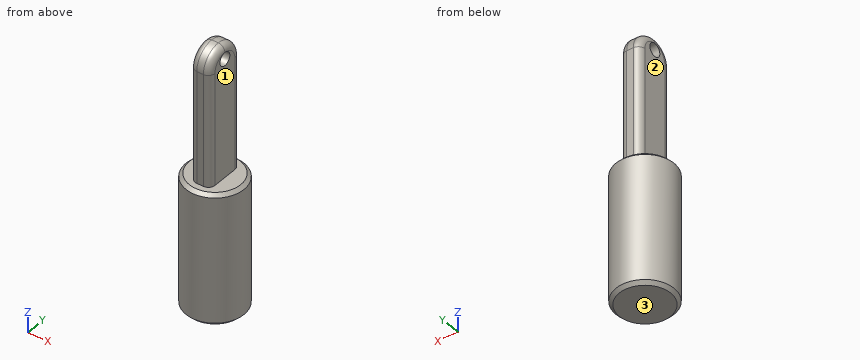
from build123d import *

# Parameters (mm, degrees)
SKETCH2_R           = 22
BOSS_EXTRUDE1_DEPTH = 100
SKETCH4_W           = 100
SKETCH4_H           = 30
BOSS_EXTRUDE2_DEPTH = 7.5
FILLET1_R           = 15
SKETCH5_R           = 5
CUT_EXTRUDE1_DEPTH  = 107.556323135
FILLET2_R           = 5
CHAMFER1_SIZE       = 2.5


with BuildPart() as part:
    # Sketch2 → Boss-Extrude1 (new body)
    with BuildSketch(Plane.XY):
        Circle(SKETCH2_R)
    extrude(amount=-BOSS_EXTRUDE1_DEPTH)

    # Sketch4 → Boss-Extrude2 (add, symmetric)
    with BuildSketch(Plane(origin=(0, 0, 0), x_dir=(0, 0, -1), z_dir=(1, 0, 0))):
        with Locations((-50, 0)):
            Rectangle(SKETCH4_W, SKETCH4_H)
    extrude(amount=BOSS_EXTRUDE2_DEPTH, both=True)

    # Fillet1
    fillet1_edges = [part.edges().sort_by_distance(p)[0] for p in [
        (0, -15, 100),
        (0, 15, 100),
    ]]
    fillet(fillet1_edges, radius=FILLET1_R - 0.0001)  # a hair under: the kernel refuses the full size

    # Sketch5 → Cut-Extrude1 (cut, through all)
    with BuildSketch(Plane(origin=(7.5, 0, 0), x_dir=(0, 0, -1), z_dir=(1, 0, 0))):
        with Locations((-90, 0)):
            Circle(SKETCH5_R)
    extrude(amount=-CUT_EXTRUDE1_DEPTH, mode=Mode.SUBTRACT)

    # Fillet2
    fillet2_edges = [part.edges().sort_by_distance(p)[0] for p in [
        (-7.5, -15, 42.50005),
        (7.5, -15, 42.50005),
        (-7.5, 10.606631007, 95.606631007),
        (-7.5, -10.606631007, 95.606631007),
        (7.5, 10.606631007, 95.606631007),
        (7.5, -10.606631007, 95.606631007),
        (-7.5, 15, 42.50005),
        (7.5, 15, 42.50005),
    ]]
    fillet(fillet2_edges, radius=FILLET2_R - 0.0001)  # a hair under: the kernel refuses the full size

    # Chamfer1
    chamfer1_edges = [part.edges().sort_by_distance(p)[0] for p in [
        (-22, 0, 0),
        (-22, 0, -100),
    ]]
    chamfer(chamfer1_edges, length=CHAMFER1_SIZE)


solid = part.part
For this review, take the finished solid that the model builds, in its own axes (mm). Face numbers are marked on the shaded views. A direction names the side the tool comes from. Give positions to 0.01 mm unless a question says otherwise; leave off trailing zeros. Order: outer loops, then holes, each group sorted by start corner. A loop starts at its lowest first (then second) coordinate and runs counter-clockwise, first axis right, second up. Notation, with made-up numbers: M 28,14 L 52,14 A9 ccw 52,26 Z; hole C -32.5,-10 d2. An arc over 180 degrees is marked long. Answer in a Markdown table with one row per item. Add a question column.
(1) For pin 1 (3 mm diameter, centred on x = -17, z = 2.5, fed in from +Y); pin 2 (13 mm diameter, centred on y = 0, z = 90, fed in from +X); pin 3 (12 mm diameter, centred on y = -4.5, z = -41.5, fed in from +X); pin 4 (4 mm diameter, centred on x = 0, z = 42, fed in from -Y), all flat-tipped, find the tip position at first contact; note any pin that passes through.
(2) Consider section B-B on z = 81. State the section outline as (x, y) points, and give its area (3 significant figures).
(3) Wall thickness on probe 1 along Y at (x, z) = (-1.5, 72); probe 2 along Z at (x, y) = (-13, 11); probe 3 along Y at (x, z) = (-3.5, 90) (3 decimals): over which ranges is each line inside the solid? List them lowest first. Write a range as [from, to].
(4) Consider section C-C on z = -66. State the section outline as (x, y) points.
(5) For the marked faces 1, 2 and 3, list the 3-axis set-ups (+Z, -Z, +X, -X, +Y, -Y) from which the entire face can be reached by the end or side of a thin tool; tool diameter is ignored.
Evaluation:
| question | item | result |
|---|---|---|
| 1 | pin 1 | passes through |
| 1 | pin 2 | stops at x = 7.5 |
| 1 | pin 3 | stops at x = 22 |
| 1 | pin 4 | stops at y = -15 |
| 2 | outline | M -7.5,-10 A5 ccw -2.5,-15 L 2.5,-15 A5 ccw 7.5,-10 L 7.5,10 A5 ccw 2.5,15 L -2.5,15 A5 ccw -7.5,10 Z |
| 2 | area | 429 mm^2 |
| 3 | probe 1 | y = [-15, 15] |
| 3 | probe 2 | z = [-100, 0] |
| 3 | probe 3 | y = [-14.035, -5], [5, 14.035] |
| 4 | outline | C 0,0 d44 |
| 5 | face 1 | +Z, +X, +Y, -Y |
| 5 | face 2 | +Z, -X, +Y, -Y |
| 5 | face 3 | -Z, +X, -X, +Y, -Y |
